Geometry check sheet. Reference: drawing and pictorial views, mm from the part's lowest x, y, z. A direction names the side the tool comes from. Round coordinates to 2 decimals unless told otherwise and drop trailing zeros. Loops run counter-clockwise (first coordinate to the right, second up) from the corner with the lowest first, then second, coordinate; pieces in that order, holes last. Notation, with made-up numbers: (37, -3) -> (74, -3) arc R13 ccw to (74, 22) -> close; hole circle Ø4 at (43, 24). An arc over 180 degrees is marked (long way). Write item = value, one per line.
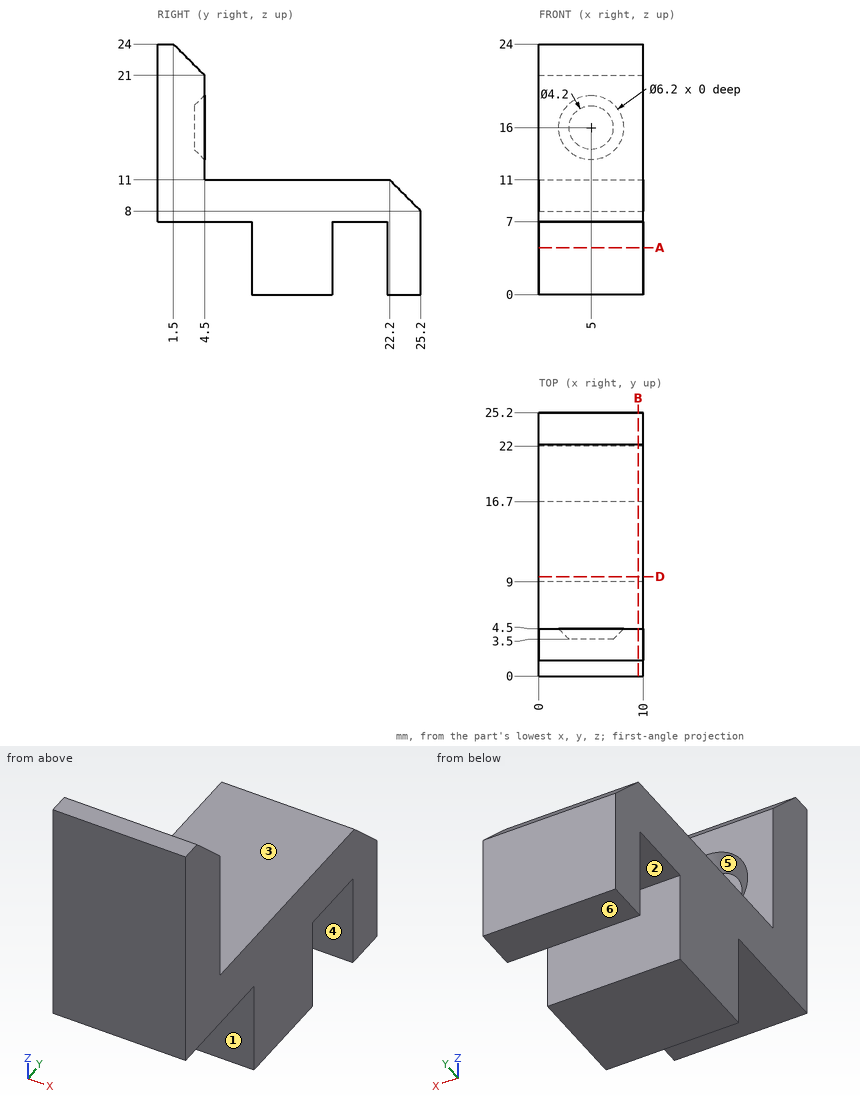
(1) Go/stop test with flat-tipped pins: pin 1 Ø3.5 at (x, z) = (6, 2) entering from -Y; pin 2 Ø2 at (x, z) = (4, 16) entering from +Y; pin 3 Ø3 at (x, z) = (4.5, 10.5) entering from +Y. Record where each tip stops, or that it passes through.
Filled sheet:
pin_1 = 9
pin_2 = 3.5
pin_3 = 24.2
(2) Sectioned sample at D-D, the plane y = 9.5. Record the cut outline in (x, z).
Filled sheet:
outline = (0, 0) -> (10, 0) -> (10, 11) -> (0, 11) -> close
(3) Material ranges on probe 1 along Y at (x, z) = (2.25, 3.75); probe 2 along Z at (x, y) = (5, 4.55); probe 3 along Y at (x, z) = (5, 17.25), recorded low to high. Write a range as from..to.
Filled sheet:
probe_1 = 9..16.7, 22..25.2
probe_2 = 7..11
probe_3 = 0..3.5
(4) Draft check along Y on the marked faces 4, 5 and 6. Enter one of: released by +Y, released by -Y, zero draft, split by the parting line, or undercut.
Filled sheet:
face_4 = undercut
face_5 = released by +Y
face_6 = zero draft
(5) Sectioned sample at B-B, the plane x = 9.5. Record the cut outline in (y, z), and give its area (3 significant figures).
Filled sheet:
outline = (0, 7) -> (9, 7) -> (9, 0) -> (16.7, 0) -> (16.7, 7) -> (22, 7) -> (22, 0) -> (25.2, 0) -> (25.2, 8) -> (22.2, 11) -> (4.5, 11) -> (4.5, 21) -> (1.5, 24) -> (0, 24) -> close
area = 227 mm2
(6) Set-up check for the marked faces 1, 2 and 3: record each of +Z, -Z, +X, -X, +Y, -Y from which the full face is reachable in a straight line by a thin tool's end or side.
Filled sheet:
face_1 = -Z, +X, -X, -Y
face_2 = -Z, +X, -X
face_3 = +Z, +X, -X, +Y
(7) Sectioned sample at A-A, the plane z = 4.5. Record the cut outline in (x, y), and give its area (3 significant figures).
Filled sheet:
outline = (0, 9) -> (10, 9) -> (10, 16.7) -> (0, 16.7) -> close; (0, 22) -> (10, 22) -> (10, 25.2) -> (0, 25.2) -> close
area = 109 mm2
